Model file for the job. Use its own axes, mm. A direction names the side the tool comes from. Round coordinates to 2 decimals unless told otherwise and drop trailing zeros. Loops run counter-clockwise (first coordinate to the right, second up) from the corner with the lowest first, then second, coordinate; pieces in that order, holes last. Notation, with made-up numbers: M -2,17 L 42,17 A29 ccw 42,42 Z; hole C 68,75 d7. An arc over 180 degrees is marked long. Use a Markdown table: item, result. Add a question column.
Item 1: Pin check, flat tips, straight feed: P1, Ø4, axis at x = 6.5, z = -59, coming from the -Y side; P2, Ø6.5, axis at x = -47.88, z = -46.47, coming from the -Y side. Stop position of each tip, or through.
Item 2: Two-plate mould, pull along Z, no slides. Class faces 1 (the cylindrical face through (-10.3, -82.5, -48.1)), 2 (the flat face through (-1, -39, -74.893)), 3 (the cylindrical face through (33.25, -82.46, 64.12)), 4 (the flat face through (-74.906, -39, -1)): +Z half, -Z half, draft (parallel to the pull), parting line (faces both ways), or undercut.
Item 3: Saw through at A-A on z = 9. Write the cut outline in (x, y), then the cut area to 3 significant figures.
Item 4: Saw through at B-B on x = -23. Write the cut outline in (y, z), then the cut area to 3 significant figures.
Item 5: Wall check: L1, parallel to Y at x = -5, z = 3.5. Give the ranges that are in metal, low to high. Write a range as from..to.
Item 6: Tool access for faces 5 (the flat face through (74.316, -39, -1)), 6 (the cylindrical face through (6.44, -82.46, -35.58)): list every direction of +Z, -Z, +X, -X, +Y, -Y with a clear straight run to the whole face (end or side of a thin tool).
```python
from build123d import *

# Parameters (mm, degrees)
F0_W     = 149.222113
F0_H     = 150.687955
F1_DEPTH = 80
F2_R     = 32.024782
F2_R_2   = 30.381377
F3_DEPTH = 5
F4_R     = 33.265998
F4_R_2   = 2.039344
F4_R_3   = 33.931955
F5_DEPTH = 5


with BuildPart() as f1:
    # F0 (on Front) → F1 (new body)
    with BuildSketch(Plane.XZ):
        with Locations((-0.295292, 0.451285)):
            Rectangle(F0_W, F0_H)
    extrude(amount=F1_DEPTH)

    # F2 (on face) → F3 (join)
    with BuildSketch(Plane.XZ.offset(80)):
        with Locations((-41.818906, 33.70855)):
            Circle(F2_R)
        with Locations((37.204407, 33.996958)):
            Circle(F2_R_2)
    extrude(amount=F3_DEPTH)

    # F4 (on face) → F5 (join)
    with BuildSketch(Plane.XZ.offset(80)):
        with Locations((-41.029103, -35.356872)):
            Circle(F4_R)
        with Locations((-47.875438, -46.468385)):
            Circle(F4_R_2, mode=Mode.SUBTRACT)
        with Locations((40.339995, -37.069906)):
            Circle(F4_R_3)
    extrude(amount=F5_DEPTH)


solid = f1.part
```
Entries:
| question | item | result |
|---|---|---|
| 1 | P1 | y = -80 |
| 1 | P2 | y = -85 |
| 2 | face 1 | undercut |
| 2 | face 2 | -Z half |
| 2 | face 3 | undercut |
| 2 | face 4 | draft |
| 3 | outline | M -74.91,-80 L -62.19,-80 L -62.19,-85 L -21.45,-85 L -21.45,-80 L 19.94,-80 L 19.94,-85 L 54.47,-85 L 54.47,-80 L 74.32,-80 L 74.32,0 L -74.91,0 Z |
| 3 | area | 12,300 mm2 |
| 4 | outline | M -85,-63.31 L -80,-63.31 L -80,-74.89 L 0,-74.89 L 0,75.8 L -80,75.8 L -80,59.62 L -85,59.62 L -85,7.8 L -80,7.8 L -80,-7.4 L -85,-7.4 Z |
| 4 | area | 12,600 mm2 |
| 5 | L1 | -80..0 |
| 6 | face 5 | +Z, -Z, +X, +Y, -Y |
| 6 | face 6 | -Y |
